Can you work these out from the model? Positions are in its coordinate system, mm. Face numbers are marked on the shaded views. A direction names the side the tool comes from. Coordinates: 2 decimals unless noted, no trailing zeros. Order: outer loops, then holes, each group sorted by start corner. A loop starts at its lowest first (then second) coordinate and runs counter-clockwise, first axis right, second up. Notation, with made-up numbers: (-17, 85.25) -> (-8, 85.25) arc R4 ccw to (-8, 89.25) -> close; hole circle Ø6 at (81, -21.5). An arc over 180 degrees is marked (long way). Answer in a Markdown table with one row per item.
```python
from build123d import *

# Parameters (mm, degrees)
SKETCH1_W           = 30
SKETCH1_H           = 30
BOSS_EXTRUDE1_DEPTH = 30
CUT_EXTRUDE1_DEPTH  = 30
CUT_EXTRUDE2_DEPTH  = 30
CUT_EXTRUDE3_DEPTH  = 30
CUT_EXTRUDE4_DEPTH  = 30
CUT_EXTRUDE5_DEPTH  = 15
SKETCH6_R           = 1.5
CUT_EXTRUDE6_DEPTH  = 10
SKETCH7_R           = 1.5
CUT_EXTRUDE7_DEPTH  = 10
SKETCH8_R           = 1.5
CUT_EXTRUDE8_DEPTH  = 10
SKETCH9_R           = 1.5
CUT_EXTRUDE9_DEPTH  = 10
SKETCH10_R          = 1.5
CUT_EXTRUDE10_DEPTH = 10
SKETCH11_R          = 1.5
CUT_EXTRUDE11_DEPTH = 10


with BuildPart() as part:
    # Sketch1 → Boss-Extrude1 (new body)
    with BuildSketch(Plane.XY):
        with Locations((15, 15)):
            Rectangle(SKETCH1_W, SKETCH1_H)
    extrude(amount=-BOSS_EXTRUDE1_DEPTH)

    # Sketch2 → Cut-Extrude1 (cut)
    with BuildSketch(Plane.XY):
        Polygon((15, 30), (30, 15), (45, 15), (45, 45.619084343), (15, 40.368332998), align=None)
    extrude(amount=-CUT_EXTRUDE1_DEPTH, mode=Mode.SUBTRACT)

    # Sketch3 → Cut-Extrude2 (cut)
    with BuildSketch(Plane.ZY):
        Polygon((0, 15), (-15, 30), (-15, 36.177250049), (9.539630377, 36.177250049), (9.539630377, 15), align=None)
    extrude(amount=-CUT_EXTRUDE2_DEPTH, mode=Mode.SUBTRACT)

    # Sketch4 → Cut-Extrude3 (cut)
    with BuildSketch(Plane.XZ):
        Polygon((15, 0), (30, -15), (40.227840819, -15), (40.227840819, 9.317096887), (15, 8.966367386), align=None)
    extrude(amount=-CUT_EXTRUDE3_DEPTH, mode=Mode.SUBTRACT)

    # 3DSketch1 → Cut-Extrude4 (cut)
    with BuildSketch(Plane(origin=(33.996909354, 3.570047518, -7.566956872), x_dir=(-0.34464530014522, 0.4926249601560642, 0.7990871452595439), z_dir=(-0.2113248654051872, 0.788675134594813, -0.5773502691896257))):
        Polygon((0, 0), (25.47550653, -16.637081723), (36.340550094, 0), (10.865043564, 16.637081723), align=None)
    extrude(amount=CUT_EXTRUDE4_DEPTH, mode=Mode.SUBTRACT)

    # Sketch5 → Cut-Extrude5 (cut)
    with BuildSketch(Plane(origin=(10, 10, 10), x_dir=(0.4082482904638628, 0.40824829046386263, -0.8164965809277264), z_dir=(0.5773502691896263, 0.5773502691896258, 0.5773502691896254))):
        Polygon((19.457058725, 2.946852636), (27.184465336, 5.017404997), (29.255017696, -2.710001614), (21.527611086, -4.780553975), align=None)
    extrude(amount=-CUT_EXTRUDE5_DEPTH, mode=Mode.SUBTRACT)

    # Sketch6 → Cut-Extrude6 (cut)
    with BuildSketch(Plane(origin=(0, 30, 0), x_dir=(1, 0, 0), z_dir=(0, 1, 0))):
        with Locations(Location((7.5, 22.5, 0), (0, 0, 270))):
            Circle(SKETCH6_R)
    extrude(amount=-CUT_EXTRUDE6_DEPTH, mode=Mode.SUBTRACT)

    # Sketch7 → Cut-Extrude7 (cut)
    with BuildSketch(Plane(origin=(0, 7.5, 7.5), x_dir=(1, 0, 0), z_dir=(0, 0.7071067811865477, 0.7071067811865475))):
        with Locations(Location((7.5, 21.213203436, 0), (0, 0, 270))):
            Circle(SKETCH7_R)
    extrude(amount=-CUT_EXTRUDE7_DEPTH, mode=Mode.SUBTRACT)

    # Sketch8 → Cut-Extrude8 (cut)
    with BuildSketch(Plane.XY):
        with Locations((7.5, 7.5)):
            Circle(SKETCH8_R)
    extrude(amount=-CUT_EXTRUDE8_DEPTH, mode=Mode.SUBTRACT)

    # Sketch9 → Cut-Extrude9 (cut)
    with BuildSketch(Plane(origin=(22.5, 22.5, 0), x_dir=(0, 0, -1), z_dir=(0.7071067811865474, 0.7071067811865477, 0))):
        with Locations(Location((22.5, -0.001601718, 0), (0, 0, 90))):
            Circle(SKETCH9_R)
    extrude(amount=-CUT_EXTRUDE9_DEPTH, mode=Mode.SUBTRACT)

    # Sketch10 → Cut-Extrude10 (cut)
    with BuildSketch(Plane(origin=(30, 0, 0), x_dir=(0, 0, -1), z_dir=(1, 0, 0))):
        with Locations(Location((22.5, 7.5, 0), (0, 0, 90))):
            Circle(SKETCH10_R)
    extrude(amount=-CUT_EXTRUDE10_DEPTH, mode=Mode.SUBTRACT)

    # Sketch11 → Cut-Extrude11 (cut)
    with BuildSketch(Plane(origin=(7.5, 0, 7.5), x_dir=(0.7071067811865475, 0, -0.7071067811865477), z_dir=(0.7071067811865477, 0, 0.7071067811865475))):
        with Locations((21.211601718, 7.5)):
            Circle(SKETCH11_R)
    extrude(amount=-CUT_EXTRUDE11_DEPTH, mode=Mode.SUBTRACT)


solid = part.part
```
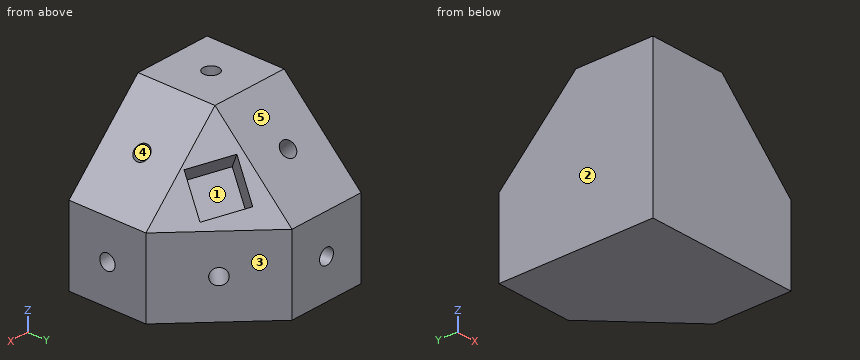
(1) Suppose I cut it at A-A (z = -2). Please give me the cut outline in (x, y), and give its area (3 significant figures).
Response values:
| item | result |
|---|---|
| outline | (0, 0) -> (17, 0) -> (17, 15) -> (15, 17) -> (0, 17) -> close; hole circle Ø3 at (7.5, 7.5) |
| area | 280 mm2 |
(2) Will these pins go through, and if not, where does the flat tip stop? pin 1 Ø1.5 at (y, z) = (8, -23) entering from +X; pin 2 Ø1.5 at (x, y) = (6, 22.5) entering from +Z.
Response values:
| item | result |
|---|---|
| pin 1 | x = 20 |
| pin 2 | z = -6.75 |
(3) I need wall thicknesses on line 1 (Y direction, x = 9.75, z = -18); line 2 (Z direction, x = 19.5, y = 20.5); line 3 (Y direction, x = 20.25, z = -16). Which ranges of each line are inside material? Lowest first, please. Write a range as [from, to].
Response values:
| item | result |
|---|---|
| line 1 | [0, 12.27], [16.12, 30] |
| line 2 | [-30, -23.82], [-21.18, -14.71] |
| line 3 | [0, 15.87], [18.46, 24.75] |
(4) We'd pull the mould along X, two halves only. Please class the marked faces 3, 4 and 5: +X half, -X half, draft (parallel to the pull), parting line (faces both ways), or undercut.
Response values:
| item | result |
|---|---|
| face 3 | +X half |
| face 4 | undercut |
| face 5 | draft |
(5) Suppose I cut it at C-C (x = 3.75). Please give me the cut outline in (y, z).
Response values:
| item | result |
|---|---|
| outline | (0, -30) -> (30, -30) -> (30, -15) -> (15, 0) -> (0, 0) -> close |
(6) On a 3-axis mill with a long thin cutter (end or side, diameter ignored), from which of +Z, -Z, +X, -X, +Y, -Y can I reach the whole of each face in a straight line? I mean the marked faces 1 and 2. Say none if no direction works.
Response values:
| item | result |
|---|---|
| face 1 | none |
| face 2 | +Z, -Z, -X, +Y, -Y |
(7) Suppose I cut it at B-B (y = 7.5). Please give me the cut outline in (x, z), and give its area (3 significant figures).
Response values:
| item | result |
|---|---|
| outline | (0, -30) -> (30, -30) -> (30, -24) -> (20, -24) -> (20, -21) -> (30, -21) -> (30, -15) -> (23.56, -8.56) -> (16.49, -15.63) -> (14.37, -13.51) -> (21.44, -6.44) -> (15, 0) -> (9, 0) -> (9, -10) -> (6, -10) -> (6, 0) -> (0, 0) -> close; hole (12.48, -15.96) -> (13.78, -17.26) -> (14.26, -15.49) -> close |
| area | 696 mm2 |
